The drawing under review shows one solid part. Ordinate dimensions are in mm from its lowest x, y, z. A direction names the side the tool comes from. Coordinates: 2 decimals unless noted, no trailing zeros. Write each loop counter-clockwise with the first axis right and the second up, starting at its lowest first coordinate (ties: lowest second). Pieces come first, ordered by that corner, then holes. Notation, with made-up numbers: (61, 84.5) - (70, 84.5) arc R26 cw to (70, 122.5) - close; hole circle Ø5 at (88.25, 52.25). An arc over 180 degrees is marked (long way). Answer as CSV lines item,"result". Start each with the question number.
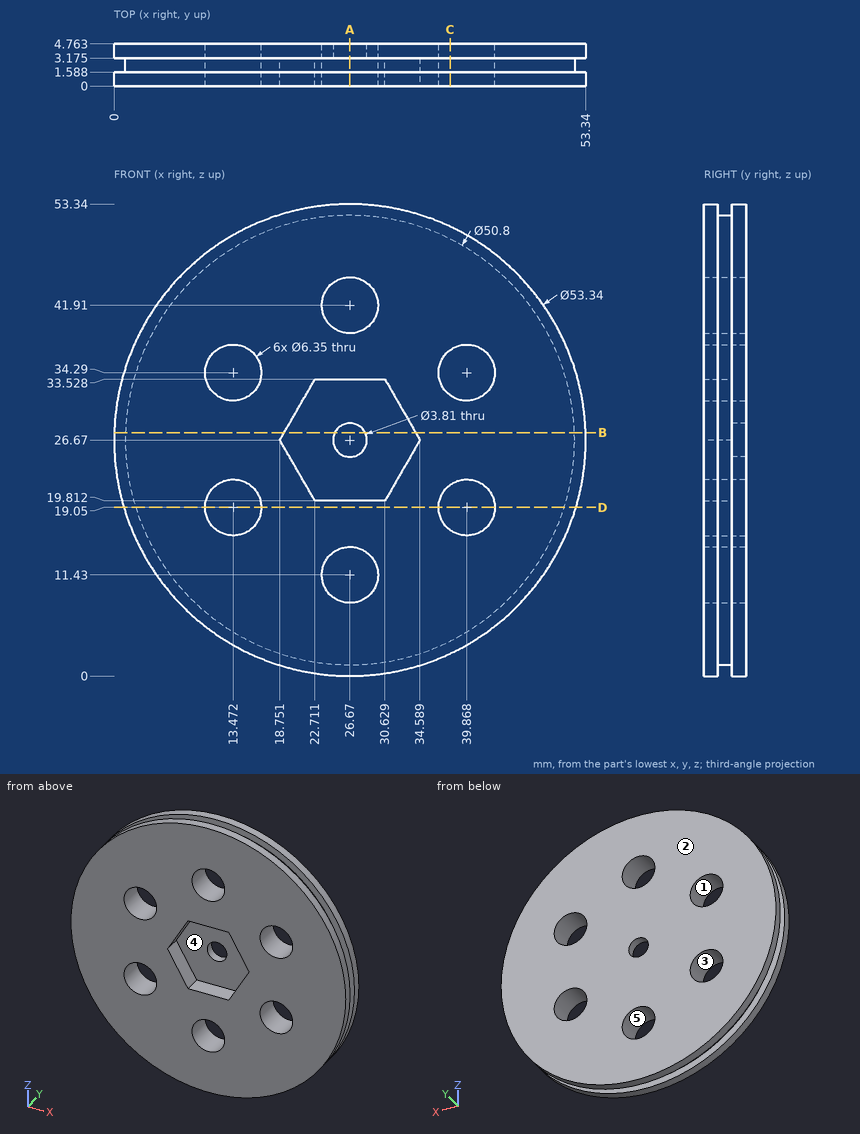
(1) For the marked faces 4 and 5, list the 3-axis set-ups (+Z, -Z, +X, -X, +Y, -Y) from which the entire face can be reached by the end or side of a thin tool; tool diameter is ignored.
(2) Add section B-B on z = 27.5. Give the boundary of the cut face in (x, y) (1 decimal), then the cut area to 3 significant figures.
(3) Wall thickness on line 1 (Z direction, x = 26.67, y = 4.3) (1 decimal); line 2 (Z direction, x = 26.67, y = 2.25) (1 decimal); line 3 (X direction, y = 1.85, z = 20.5) (1 decimal): over which ranges is each line inside the solid? List them lowest first.
(4) The part is to be moulded in two halves that separate along X. For the marked faces 1, 2 and 3, say which applies: released by +X, released by -X, zero draft, split by the parting line, or undercut.
(5) Add section D-D on z = 19.05. Give the boundary of the cut face in (x, y) (1 decimal).
(6) For pin 1 (4 mm diameter, centred on x = 26.67, z = 41.91, fed in from +Y); pin 2 (2 mm diameter, centred on x = 33, y = 1, fed in from -Z); pin 3 (1 mm diameter, centred on y = 1.5, z = 36, fed in from -X) (1 decimal); pin 4 (2 mm diameter, centred on x = 29.5, y = 1, fed in from -Z), all flat-tipped, find the tip position at first contact; note any pin that passes through.
(7) Add section A-A on x = 26.67. Give the boundary of the cut face in (y, z) (1 decimal), then the cut area to 3 significant figures.
(8) Add section C-C on x = 38. Give the boundary of the cut face in (y, z) (1 decimal).
Reported:
1,face 4,"-Y"
1,face 5,"+Y, -Y"
2,outline,"(0, 0) - (19.2, 0) - (19.2, 3.2) - (25, 3.2) - (25, 4.8) - (0, 4.8) - (0, 3.2) - (1.3, 3.2) - (1.3, 1.6) - (0, 1.6) - close; (28.4, 3.2) - (34.1, 3.2) - (34.1, 0) - (53.3, 0) - (53.3, 1.6) - (52.1, 1.6) - (52.1, 3.2) - (53.3, 3.2) - (53.3, 4.8) - (28.4, 4.8) - close"
2,area,"197 mm²"
3,line 1,"0 to 8.3, 14.6 to 24.8, 28.6 to 38.7, 45.1 to 53.3"
3,line 2,"1.3 to 8.3, 14.6 to 19.8, 33.5 to 38.7, 45.1 to 52.1"
3,line 3,"2 to 10.6, 16.3 to 22.3, 31 to 37, 42.7 to 51.3"
4,face 1,"undercut"
4,face 2,"zero draft"
4,face 3,"undercut"
5,outline,"(1.1, 0) - (10.3, 0) - (10.3, 4.8) - (1.1, 4.8) - (1.1, 3.2) - (2.4, 3.2) - (2.4, 1.6) - (1.1, 1.6) - close; (16.6, 0) - (36.7, 0) - (36.7, 4.8) - (16.6, 4.8) - close; (43, 0) - (52.2, 0) - (52.2, 1.6) - (50.9, 1.6) - (50.9, 3.2) - (52.2, 3.2) - (52.2, 4.8) - (43, 4.8) - close"
6,pin 1,"through"
6,pin 2,"z = 0.54"
6,pin 3,"x = 1.5"
6,pin 4,"z = 0.06"
7,outline,"(0, 0) - (1.6, 0) - (1.6, 1.3) - (3.2, 1.3) - (3.2, 0) - (4.8, 0) - (4.8, 8.3) - (0, 8.3) - close; (0, 14.6) - (4.8, 14.6) - (4.8, 24.8) - (3.2, 24.8) - (3.2, 19.8) - (0, 19.8) - close; (0, 33.5) - (3.2, 33.5) - (3.2, 28.6) - (4.8, 28.6) - (4.8, 38.7) - (0, 38.7) - close; (0, 45.1) - (4.8, 45.1) - (4.8, 53.3) - (3.2, 53.3) - (3.2, 52.1) - (1.6, 52.1) - (1.6, 53.3) - (0, 53.3) - close"
7,area,"140 mm²"
8,outline,"(0, 2.5) - (1.6, 2.5) - (1.6, 3.9) - (3.2, 3.9) - (3.2, 2.5) - (4.8, 2.5) - (4.8, 16.5) - (0, 16.5) - close; (0, 21.6) - (4.8, 21.6) - (4.8, 31.7) - (0, 31.7) - close; (0, 36.9) - (4.8, 36.9) - (4.8, 50.8) - (3.2, 50.8) - (3.2, 49.4) - (1.6, 49.4) - (1.6, 50.8) - (0, 50.8) - close"
